Autodesk Inventor part; units mm, degrees
ref_plane "YZ Plane" through (0, 0, 0) normal (1, 0, 0) x (0, 1, 0)
ref_plane "XZ Plane" through (0, 0, 0) normal (0, 1, 0) x (-1, 0, 0)
ref_plane "XY Plane" through (0, 0, 0) normal (0, 0, 1) x (1, 0, 0)
sketch "Sketch1" plane through (0, 0, 0) normal (0, 0, 1) x (1, 0, 0)
  line L0 (0, 0) -> (0, 350)
  line L1 (0, 350) -> (450, 350)
  line L2 (450, 350) -> (450, 0)
  line L3 (450, 0) -> (0, 0)
  line L4 (0, 0) -> (225, 0)
  line L5 (225, 350) -> (220, 350)
  line L6 (225, 350) -> (220, 350)
  line L7 (220, 350) -> (230, 350)
  line L8 (230, 350) -> (230, 0)
  line L9 (220, 350) -> (220, 0)
  line L10 (220, 0) -> (195, 0)
  line L11 (230, 0) -> (255, 0)
  line L12 (255, 0) -> (450, 350)
  line L13 (195, 0) -> (0, 350)
  line L14 (255, 0) -> (265, 0)
  line L15 (265, 0) -> (450, 332.0513)
  line L16 (195, 0) -> (185, 0)
  line L17 (185, 0) -> (0, 332.0513)
  line L18 (0, 332.0513) -> (0, 350)
  line L19 (450, 332.0513) -> (450, 350)
extrude "Extrusion1" add sketch "Sketch1" along normal blind 250 contours L0 L13 L3 L17 | L1 L8 L3 L9 | L2 L15 L3 L12
sketch "Sketch2" plane through (0, 0, 250) normal (0, 0, 1) x (1, 0, 0)
  line L0 (0, 350) -> (0, 332.0513)
  line L1 (450, 332.0513) -> (450, 350)
  line L2 (0, 350) -> (450, 350)
  line L3 (450, 350) -> (450, 332.0513)
  line L4 (255, 0) -> (265, 0)
  line L5 (450, 332.0513) -> (265, 0)
  line L6 (185, 0) -> (195, 0)
  line L7 (265, 0) -> (185, 0)
  line L8 (185, 0) -> (0, 332.0513)
  line L9 (0, 332.0513) -> (0, 350)
  point P0 (0, 0)
extrude "Extrusion2" add sketch "Sketch2" along normal blind 5
sketch "Sketch3" plane through (0, 0, 0) normal (0, 0, -1) x (-1, 0, 0)
  line L0 (-450, 332.0513) -> (-450, 350)
  line L1 (-195, 0) -> (0, 350)
  line L2 (-450, 350) -> (0, 350)
  line L3 (0, 350) -> (0, 332.0513)
  line L4 (0, 350) -> (0, 332.0513)
  line L5 (0, 332.0513) -> (-185, 0)
  line L6 (0, 332.0513) -> (-185, 0)
  line L7 (-185, 0) -> (-265, 0)
  line L8 (-265, 0) -> (-450, 332.0513)
  line L9 (-265, 0) -> (-450, 332.0513)
  line L10 (-450, 332.0513) -> (-450, 350)
  point P0 (0, 0)
extrude "Extrusion3" add sketch "Sketch3" along normal blind 5
fillet "Fillet1" radius 2 1 edges at (255, 0, 125)
fillet "Fillet2" radius 2 1 edges at (230, 0, 125)
fillet "Fillet3" radius 2 1 edges at (220, 0, 125)
fillet "Fillet4" radius 2 1 edges at (195, 0, 125)
sketch "Sketch4" plane through (0, 332.0513, 255) normal (-1, 0, 0) x (0, 0, 1)
  line L0 (-255, 17.9487) -> (-260, 17.9487)
  line L1 (-260, 17.9487) -> (-260, 8.9744)
  line L2 (-260, 17.9487) -> (-260, 0)
  line L3 (-1.0875, 8.9744) -> (-260, 8.9744)
  line L4 (-5, 17.9487) -> (-5, -330.0513)
  line L5 (-260, 8.9744) -> (-135, 8.9744)
  circle A0 centre (-135, 8.9744) radius 5
  point P0 (-255, -332.0513)
  dimension "d20" = 125
  dimension "d21" = 10
extrude "Extrusion4" cut sketch "Sketch4" against normal blind 10
sketch "Sketch5" plane through (450, 332.0513, 255) normal (1, 0, 0) x (0, 0, -1)
  circle A0 centre (135, 8.9744) radius 5
  point P0 (255, -332.0513)
extrude "Extrusion5" cut sketch "Sketch5" against normal blind 10
sketch "Sketch6" plane through (0, 332.0513, 255) normal (-1, 0, 0) x (0, 0, 1)
  circle A0 centre (-135, 8.9744) radius 5
  circle A1 centre (-210, 8.9744) radius 5
  circle A2 centre (-50.1609, 8.9744) radius 5
  point P0 (-255, -332.0513)
extrude "Extrusion6" cut sketch "Sketch6" against normal blind 10 contours A1 | A2
sketch "Sketch7" plane through (450, 332.0513, 255) normal (1, 0, 0) x (0, 0, -1)
  line L0 (5, 17.9487) -> (0, 17.9487)
  line L1 (5, 17.9487) -> (5, 8.9487)
  line L2 (5, 17.9487) -> (5, -329.0779)
  circle A0 centre (50.1609, 8.9744) radius 5
  line L3 (5, 8.9487) -> (50.1609, 8.9744)
  circle A1 centre (210, 8.9744) radius 5
  circle A2 centre (210, 8.9744) radius 5
  point P0 (255, -332.0513)
  dimension "d40" = 9
extrude "Extrusion7" cut sketch "Sketch7" against normal blind 10 contours A1
sketch "Sketch8" plane through (450, 332.0513, 255) normal (1, 0, 0) x (0, 0, -1)
  circle A0 centre (50.1609, 8.9744) radius 5
  circle A1 centre (50.1609, 8.9744) radius 5
  point P0 (255, -332.0513)
extrude "Extrusion8" cut sketch "Sketch8" against normal blind 10
sketch "Sketch9" plane through (185, 0, 255) normal (0, -1, 0) x (1, 0, 0)
  line L0 (-185, -260) -> (-185, 0)
  line L1 (265, -260) -> (-185, -260)
  line L2 (-185, -260) -> (-185, 0)
  line L3 (-185, 0) -> (265, 0)
  line L4 (265, 0) -> (265, -260)
  point P0 (-185, -255)
extrude "Extrusion9" add sketch "Sketch9" along normal blind 12
sketch "Sketch10" plane through (185, -12, 255) normal (0, -1, 0) x (1, 0, 0)
  line L0 (35, -5) -> (35, -255)
  line L1 (14.5122, -257.9685) -> (35, -257.9685)
  line L2 (35, -257.9685) -> (35, -5)
  line L3 (35, -5) -> (14.5122, -5)
  line L4 (14.5122, -5) -> (14.5122, -257.9685)
  point P0 (-185, -255)
extrude "Extrusion10" cut sketch "Sketch10" against normal blind 12
sketch "Sketch11" plane through (185, 0, 255) normal (0, 1, 0) x (1, 0, 0)
  line L0 (73.4037, 255) -> (43, 255)
  line L1 (45.375, 255) -> (71.2984, 255)
  line L2 (71.2984, 255) -> (71.2984, 5.0453)
  line L3 (71.2984, 5.0453) -> (45.375, 5.0453)
  line L4 (45.375, 5.0453) -> (45.375, 255)
  point P0 (-185, 255)
extrude "Extrusion11" cut sketch "Sketch11" against normal blind 12
sketch "Sketch12" plane through (450, 0, 255) normal (1, 0, 0) x (0, 0, -1)
  circle A0 centre (50.1609, -6.6697) radius 2.5
  circle A1 centre (211.0368, -6.6697) radius 2.5
  point P0 (255, 0)
extrude "Extrusion12" cut sketch "Sketch12" against normal blind 10 contours A1
sketch "Sketch13" plane through (450, 0, 255) normal (1, 0, 0) x (0, 0, -1)
  circle A0 centre (49.8818, -6) radius 2.5
  point P0 (255, 0)
extrude "Extrusion13" cut sketch "Sketch13" against normal blind 25
sketch "Sketch14" plane through (0, 0, -5) normal (-1, 0, 0) x (0, 0, 1)
  circle A0 centre (48.9632, -6.6697) radius 2.5
  point P0 (5, 0)
extrude "Extrusion14" cut sketch "Sketch14" against normal blind 25
sketch "Sketch15" plane through (0, 0, -5) normal (-1, 0, 0) x (0, 0, 1)
  circle A0 centre (209.8391, 341.0256) radius 5
  circle A1 centre (210.1182, -6) radius 2.5
  circle A2 centre (210.1182, -6) radius 2.5
  point P0 (5, 0)
extrude "Extrusion15" cut sketch "Sketch15" against normal blind 25 contours A1
sketch "Sketch16" plane through (0, 0, 255) normal (0, 0, 1) x (1, 0, 0)
  circle A0 centre (175, -8) radius 2.5
  circle A1 centre (325, -8) radius 2.5
  point P0 (0, 0)
extrude "Extrusion16" cut sketch "Sketch16" against normal blind 25
sketch "Sketch17" plane through (0, 0, -5) normal (0, 0, -1) x (-1, 0, 0)
  line L0 (0, 0) -> (0, -8)
  circle A0 centre (-175, -8) radius 2.5
  circle A1 centre (-325, -8) radius 2.5
extrude "Extrusion17" cut sketch "Sketch17" against normal blind 25
sketch "Sketch18" plane through (0, 0, 255) normal (0, 0, 1) x (1, 0, 0)
  circle A0 centre (275.1205, -8.1253) radius 2.5
  point P0 (0, 0)
extrude "Extrusion18" cut sketch "Sketch18" against normal blind 25
sketch "Sketch19" plane through (0, 0, -5) normal (0, 0, -1) x (-1, 0, 0)
  line L0 (-175.0524, -7.9196) -> (-275.0524, -7.9196)
  circle A0 centre (-275.0524, -7.9196) radius 2.5
  point P0 (0, 0)
  dimension "d85" = 100
  dimension "d86" = 5
extrude "Extrusion19" cut sketch "Sketch19" against normal blind 25
sketch "Sketch20" plane through (0, 0, 255) normal (0, 0, 1) x (1, 0, 0)
  line L0 (0, 0) -> (0, -4.6382)
  circle A0 centre (75, -4.6382) radius 2.5
  line L1 (450, 0) -> (265, 0)
  line L2 (450, 0) -> (450, -6)
  line L3 (450, 0) -> (450, -12)
  circle A1 centre (375, -6) radius 2.5
extrude "Extrusion20" cut sketch "Sketch20" against normal blind 25
sketch "Sketch21" plane through (450, 0, 255) normal (1, 0, 0) x (0, 0, -1)
  circle A0 centre (75, -5.6253) radius 2.5
  circle A1 centre (185, -6) radius 2.5
  point P0 (255, 0)
extrude "Extrusion21" cut sketch "Sketch21" against normal blind 25
sketch "Sketch22" plane through (0, 0, -5) normal (-1, 0, 0) x (0, 0, 1)
  circle A0 centre (75, -6) radius 2.5
  line L0 (260, 0) -> (260, -12)
  circle A1 centre (185, -5.9997) radius 2.5
  point P0 (5, 0)
extrude "Extrusion22" cut sketch "Sketch22" against normal blind 25
properties part number "new container"
Work out the finished part from the listing and answer in its coordinate system (mm). A direction names the side the tool comes from. Round coordinates to 2 decimals unless told otherwise and drop trailing zeros. Loops run counter-clockwise (first coordinate to the right, second up) from the corner with the lowest first, then second, coordinate; pieces in that order, holes last. Notation, with made-up numbers: (70, 13.5) -> (128, 13.5) arc R19 cw to (128, 31.5) -> close; hole circle Ø9 at (68, -3.75). An arc over 180 degrees is marked (long way). Use one line per item in the form item = value.
(1) Find section B-B on x = 61.5. Give the vertices of the cut face in (y, z).
Answer list:
outline = (-12, -5) -> (0, -5) -> (0, 255) -> (-12, 255) -> close; (221.67, -5) -> (350, -5) -> (350, 0) -> (239.62, 0) -> (239.62, 250) -> (350, 250) -> (350, 255) -> (221.67, 255) -> close
(2) For a pull along Y with two mould halves and no side action, classify faces 6 (the flat face through (91, 0, 127)), 7 (the flat face through (316, 212, 0)) as released by +Y, released by -Y, zero draft, split by the parting line, or undercut.
Answer list:
face_6 = undercut
face_7 = zero draft
(3) Find section A-A on y = 77. Give the vertices of the cut face in (x, z).
Answer list:
outline = (142.1, -5) -> (307.9, -5) -> (307.9, 255) -> (142.1, 255) -> close; hole (152.1, 0) -> (220, 0) -> (220, 250) -> (152.1, 250) -> close; hole (230, 0) -> (297.9, 0) -> (297.9, 250) -> (230, 250) -> close
(4) Straight lines are drawn through the part: line 1 (Y direction, x = 5, z = 45); line 2 (X direction, y = 17.5, z = 243.5); line 3 (X direction, y = 96, z = 21). For each, find the intervals that lie inside material, in ascending order.
Answer list:
line_1 = -12 to -8.94, -4.39 to 0, 323.08 to 336.03
line_2 = 175.25 to 185.25, 220 to 230, 264.75 to 274.75
line_3 = 131.51 to 141.51, 220 to 230, 308.49 to 318.49
(5) A tool of negligible diameter and unlimited length cuts with its end or side. For faces 1 (the flat face through (210, -6, -2.968)), 2 (the flat face through (220, 178, 123)), 3 (the flat face through (230, 0, 126)), 4 (the cylindrical face through (2.977, 336.145, 203.755)), 5 (the flat face through (137, 207, 250)), from which of +Z, -Z, +X, -X, +Y, -Y can it reach the whole face along a straight path? Write none if from no direction.
Answer list:
face_1 = -Y
face_2 = +Y, -Y
face_3 = none
face_4 = -X
face_5 = +Y
(6) Flat-ended cylindrical pins translate along their axes: P1, Ø1.5, axis at y = 296, z = 134.5, coming from the -X side; P2, Ø1, axis at y = 204, z = 196, coming from the +X side; P3, Ø4, axis at y = 40, z = 89, coming from the +X side; P4, Ø13, axis at y = -4.5, z = 152.5, coming from the -X side. Find the tip coordinate at first contact, or state that the pin passes through.
Answer list:
P1 = 19.67
P2 = 378.94
P3 = 288.4
P4 = 0
(7) Find section C-C on y = 220.5. Give the vertices of the cut face in (x, z).
Answer list:
outline = (62.15, -5) -> (387.85, -5) -> (387.85, 255) -> (62.15, 255) -> close; hole (72.15, 0) -> (220, 0) -> (220, 250) -> (72.15, 250) -> close; hole (230, 0) -> (377.85, 0) -> (377.85, 250) -> (230, 250) -> close
